Here's how the part is built. I have some questions about the finished solid (model axes, mm). Coordinates: 2 decimals unless noted, no trailing zeros. Write each loop counter-clockwise with the first axis right and the second up, starting at its lowest first coordinate (ties: lowest second). Pieces come first, ordered by that corner, then holes.
Item 1: If we section it at C-C (y = 10.5): Please give me the cut outline in (x, z).
Item 2: If we section it at A-A (x = -15.5): Please give me the cut outline in (y, z).
Item 3: If we section it at B-B (y = 19): Please give me the cut outline in (x, z).
Item 4: If I drill on line 1 (Z direction, x = -8, y = -17.5); line 2 (Z direction, x = 20, y = 8); line 3 (Y direction, x = -6.5, z = 128), over which ranges is the centre line in solid material (lowest first)?
from build123d import *

# Parameters (mm, degrees)
SKETCH1_W               = 45
SKETCH1_H               = 45
BOSS_EXTRUDE1_DEPTH     = 138
CUT_EXTRUDE1_DEPTH      = 23.5
CUT_EXTRUDE1_DEPTH_BACK = 23.5


with BuildPart() as part:
    # Sketch1 → Boss-Extrude1 (new body)
    with BuildSketch(Plane.XY):
        Rectangle(SKETCH1_W, SKETCH1_H)
    extrude(amount=BOSS_EXTRUDE1_DEPTH)

    # Sketch2 → Cut-Extrude1 (cut, two sides)
    with BuildSketch(Plane(origin=(0, 0, 0), x_dir=(0, 0, -1), z_dir=(1, 0, 0))) as cut_extrude1_sk:
        with BuildLine():
            Line((-138, 22.5), (-138, 0))
            ThreePointArc((-138, 0), (-131.409902577, 15.909902577), (-115.5, 22.5))
            Line((-115.5, 22.5), (-138, 22.5))
        make_face()
        with BuildLine():
            Line((-138, -22.5), (-115.5, -22.5))
            ThreePointArc((-115.5, -22.5), (-131.409902577, -15.909902577), (-138, 0))
            Line((-138, 0), (-138, -22.5))
        make_face()
    extrude(amount=CUT_EXTRUDE1_DEPTH, mode=Mode.SUBTRACT)
    extrude(cut_extrude1_sk.sketch, amount=-CUT_EXTRUDE1_DEPTH_BACK, mode=Mode.SUBTRACT)


solid = part.part
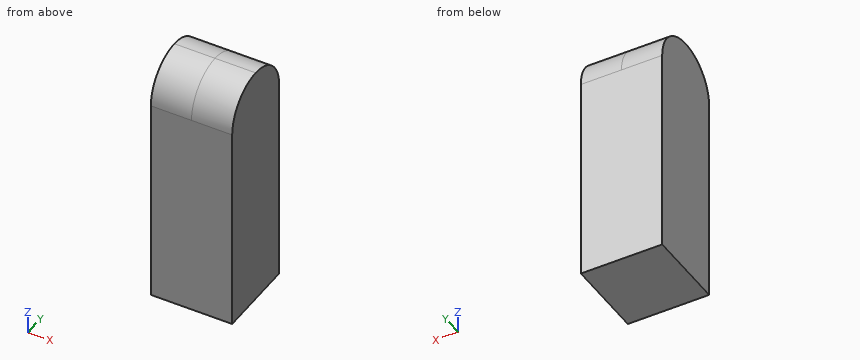
Answer list:
1. outline: (-22.5, 0) - (22.5, 0) - (22.5, 135.4) - (-22.5, 135.4) - close
2. outline: (-22.5, 0) - (22.5, 0) - (22.5, 115.5) arc R22.5 ccw to (-22.5, 115.5) - close
3. outline: (-22.5, 0) - (22.5, 0) - (22.5, 127.55) - (-22.5, 127.55) - close
4. line 1: z = 0 to 129.64
4. line 2: z = 0 to 136.53
4. line 3: y = -18.71 to 18.71
